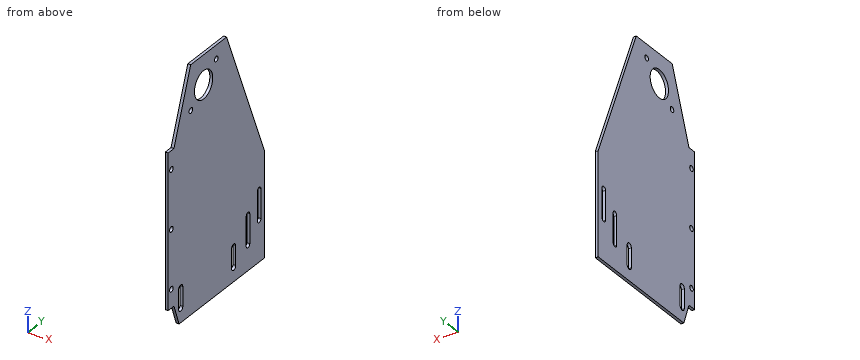
```python
from build123d import *

# Parameters (mm, degrees)
SKETCH1_W           = 300
SKETCH1_H           = 150
SKETCH1_R           = 14.235
BOSS_EXTRUDE1_DEPTH = 3
CUT_EXTRUDE1_REACH  = 5
SKETCH2_R           = 3.225
SKETCH3_R           = 2.75
CUT_EXTRUDE2_DEPTH  = 4
CUT_EXTRUDE3_DEPTH  = 4
CUT_EXTRUDE4_DEPTH  = 10
CUT_EXTRUDE5_DEPTH  = 10
SKETCH7_R           = 2.75
CUT_EXTRUDE6_DEPTH  = 4
CUT_EXTRUDE7_DEPTH  = 10


with BuildPart() as part:
    # Sketch1 → Boss-Extrude1 (new body)
    with BuildSketch(Plane(origin=(0, 0, 0), x_dir=(0, 0, -1), z_dir=(1, 0, 0))):
        with Locations((150, 75)):
            Rectangle(SKETCH1_W, SKETCH1_H)
        with Locations((30, 55)):
            Circle(SKETCH1_R, mode=Mode.SUBTRACT)
    extrude(amount=BOSS_EXTRUDE1_DEPTH)

    # Sketch2 → Cut-Extrude1 (cut, up to next)
    with BuildSketch(Plane.ZY, mode=Mode.PRIVATE) as cut_extrude1_sk1:
        with Locations((-10, 110)):
            Circle(SKETCH2_R)
    cut_extrude1_tool1 = extrude(cut_extrude1_sk1.sketch, amount=-CUT_EXTRUDE1_REACH, mode=Mode.PRIVATE) & part.part
    add(cut_extrude1_tool1.solids().sort_by_distance((0, 110, -10))[0], mode=Mode.SUBTRACT)
    # Sketch2 → Cut-Extrude1 (cut, up to next)
    with BuildSketch(Plane.ZY, mode=Mode.PRIVATE) as cut_extrude1_sk2:
        with BuildLine():
            Line((-216, 98.478413591), (-236, 98.478413591))
            ThreePointArc((-236, 98.478413591), (-239.23, 101.708413591), (-236, 104.938413591))
            Line((-236, 104.938413591), (-216, 104.938413591))
            ThreePointArc((-216, 104.938413591), (-212.77, 101.708413591), (-216, 98.478413591))
        make_face()
    cut_extrude1_tool2 = extrude(cut_extrude1_sk2.sketch, amount=-CUT_EXTRUDE1_REACH, mode=Mode.PRIVATE) & part.part
    add(cut_extrude1_tool2.solids().sort_by_distance((0, 101.708414, -226))[0], mode=Mode.SUBTRACT)
    # Sketch2 → Cut-Extrude1 (cut, up to next)
    with BuildSketch(Plane.ZY, mode=Mode.PRIVATE) as cut_extrude1_sk3:
        with BuildLine():
            Line((-236, 22.681694356), (-216, 22.681694356))
            ThreePointArc((-216, 22.681694356), (-212.775, 19.456694356), (-216, 16.231694356))
            Line((-216, 16.231694356), (-236, 16.231694356))
            ThreePointArc((-236, 16.231694356), (-239.225, 19.456694356), (-236, 22.681694356))
        make_face()
    cut_extrude1_tool3 = extrude(cut_extrude1_sk3.sketch, amount=-CUT_EXTRUDE1_REACH, mode=Mode.PRIVATE) & part.part
    add(cut_extrude1_tool3.solids().sort_by_distance((0, 19.456694, -226))[0], mode=Mode.SUBTRACT)

    # Sketch3 → Cut-Extrude2 (cut, through all)
    with BuildSketch(Plane(origin=(3, 0, 0), x_dir=(0, 0, -1), z_dir=(1, 0, 0))):
        with Locations((14.005743185, 74.73179538)):
            Circle(SKETCH3_R)
        with Locations((45.994256815, 35.26820462)):
            Circle(SKETCH3_R)
    extrude(amount=-CUT_EXTRUDE2_DEPTH, mode=Mode.SUBTRACT)

    # Sketch4 → Cut-Extrude3 (cut, through all)
    with BuildSketch(Plane(origin=(3, 0, 0), x_dir=(0, 0, -1), z_dir=(1, 0, 0))):
        Polygon((71, 9), (0, 35), (0, 0), (71, 0), align=None)
    extrude(amount=-CUT_EXTRUDE3_DEPTH, mode=Mode.SUBTRACT)

    # Sketch5 → Cut-Extrude4 (cut)
    with BuildSketch(Plane(origin=(3, 0, 0), x_dir=(0, 0, -1), z_dir=(1, 0, 0))):
        Polygon((228.92403237, 9), (250.717958721, 16.875947155), (250.717958721, 150), (312.660420977, 150), (312.660420977, -2.829604392), (228.92403237, 0), align=None)
    extrude(amount=-CUT_EXTRUDE4_DEPTH, mode=Mode.SUBTRACT)

    # Sketch6 → Cut-Extrude5 (cut)
    with BuildSketch(Plane(origin=(3, 0, 0), x_dir=(0, 0, -1), z_dir=(1, 0, 0))):
        Polygon((146.165756513, 150.745674322), (0, 90.796268719), (-32.55366639, 170.167051921), align=None)
    extrude(amount=-CUT_EXTRUDE5_DEPTH, mode=Mode.SUBTRACT)

    # Sketch7 → Cut-Extrude6 (cut, through all)
    with BuildSketch(Plane.ZY):
        with Locations((-209.962016185, 5)):
            Circle(SKETCH7_R)
        with Locations((-149.962016185, 5)):
            Circle(SKETCH7_R)
        with Locations((-89.962016185, 5)):
            Circle(SKETCH7_R)
    extrude(amount=-CUT_EXTRUDE6_DEPTH, mode=Mode.SUBTRACT)

    # Sketch8 → Cut-Extrude7 (cut)
    with BuildSketch(Plane.ZY):
        with BuildLine():
            Line((-208.485850147, 144.07811147), (-178.485850147, 144.07811147))
            ThreePointArc((-178.485850147, 144.07811147), (-175.735850147, 141.32811147), (-178.485850147, 138.57811147))
            Line((-178.485850147, 138.57811147), (-208.485850147, 138.57811147))
            ThreePointArc((-208.485850147, 138.57811147), (-211.235850147, 141.32811147), (-208.485850147, 144.07811147))
        make_face()
        with BuildLine():
            Line((-224.982842506, 126.75), (-194.982842506, 126.75))
            ThreePointArc((-194.982842506, 126.75), (-192.232842506, 124), (-194.982842506, 121.25))
            Line((-194.982842506, 121.25), (-224.982842506, 121.25))
            ThreePointArc((-224.982842506, 121.25), (-227.732842506, 124), (-224.982842506, 126.75))
        make_face()
    extrude(amount=-CUT_EXTRUDE7_DEPTH, mode=Mode.SUBTRACT)


solid = part.part
```
Could you check a few things on this model? Use its own coordinates, in mm. Round coordinates to 2 decimals unless told otherwise and drop trailing zeros. Write each loop counter-clockwise with the first axis right and the second up, starting at its lowest first coordinate (ties: lowest second). Pieces come first, ordered by that corner, then holes.
(1) For pin 1 (2 mm diameter, centred on y = 22.5, z = -125.5, fed in from -X); pin 2 (0.9 mm diameter, centred on x = 2, y = 3.5, fed in from -Z), each with a flat end and sliding along its axis, tell me the tip position at first contact or that it passes through.
Findings below:
pin 1: stops at x = 0
pin 2: stops at z = -228.92
(2) If I drill on probe 1 along Y at (x, z) = (2.75, -211.5); probe 2 along Y at (x, z) = (0.65, -210); probe 3 along Y at (x, z) = (1.55, -30) (3 decimals), over which ranges is the centre line in solid material (lowest first)?
Findings below:
probe 1: y = 0 to 2.72, 7.28 to 121.25, 126.75 to 150
probe 2: y = 0 to 2.25, 7.75 to 121.25, 126.75 to 139.03, 143.62 to 150
probe 3: y = 24.014 to 40.765, 69.235 to 103.101
(3) Suppose I cut it at D-D on x = 1.6. State how many separate pieces and enclosed holes the cut face has, and give its area (3 significant figures).
Findings below:
separate pieces: 1
enclosed holes: 10
area: 30,000 mm2
(4) Suppose I cut it at C-C on z = -32.5. Write out the boundary of the cut face in (x, y), and give its area (3 significant figures).
Findings below:
outline: (0, 23.1) - (3, 23.1) - (3, 40.99) - (0, 40.99) - close; (0, 69.01) - (3, 69.01) - (3, 104.13) - (0, 104.13) - close
area: 159 mm2
(5) Suppose I cut it at A-A on z = -204.5. Write out the boundary of the cut face in (x, y).
Findings below:
outline: (0, 0) - (3, 0) - (3, 121.25) - (0, 121.25) - close; (0, 126.75) - (3, 126.75) - (3, 138.58) - (0, 138.58) - close; (0, 144.08) - (3, 144.08) - (3, 150) - (0, 150) - close
(6) Suppose I cut it at B-B on y = 5. Write out the boundary of the cut face in (x, z).
Findings below:
outline: (0, -228.92) - (3, -228.92) - (3, -212.71) - (0, -212.71) - close; (0, -207.21) - (3, -207.21) - (3, -152.71) - (0, -152.71) - close; (0, -147.21) - (3, -147.21) - (3, -92.71) - (0, -92.71) - close; (0, -87.21) - (3, -87.21) - (3, -71) - (0, -71) - close
